Verification items for the finished model (mm, model axes). Face numbers are marked on the shaded views. A direction names the side the tool comes from. Coordinates: 2 decimals unless noted, no trailing zeros. Order: outer loops, then holes, each group sorted by start corner. A loop starts at its lowest first (then second) coordinate and runs counter-clockwise, first axis right, second up. Notation, with made-up numbers: M -2,-7.5 L 31,-7.5 A12 ccw 31,-1.5 Z; hole C 70,10.25 d8. An arc over 180 degrees is marked long. Write item = value, one per line.
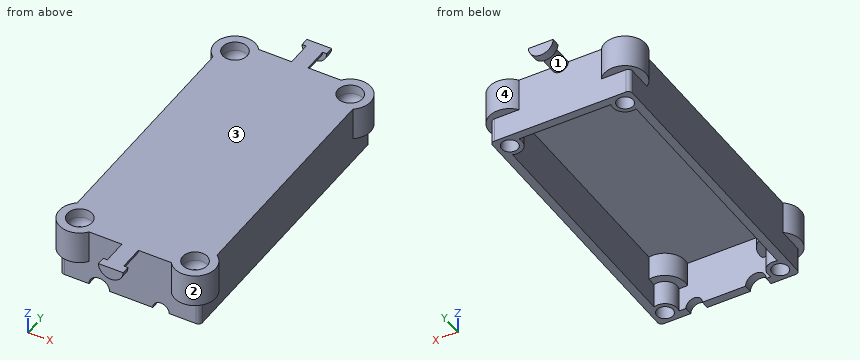
```python
from build123d import *

# Parameters (mm, degrees)
SKETCH1_W           = 34
SKETCH1_H           = 70
BOSS_EXTRUDE1_DEPTH = 14
SKETCH2_W           = 30
SKETCH2_H           = 66
CUT_EXTRUDE1_DEPTH  = 12
SKETCH3_R           = 3
BOSS_EXTRUDE2_DEPTH = 12
SKETCH4_R           = 2
CUT_EXTRUDE2_DEPTH  = 80.069589603
CUT_EXTRUDE4_REACH  = 81.07
SKETCH6_R           = 2.5
SKETCH6_R_2         = 2
FILLET1_R           = 1
BOSS_EXTRUDE3_START = -8
SKETCH7_R           = 5
SKETCH7_R_2         = 3
BOSS_EXTRUDE3_DEPTH = 8
CUT_EXTRUDE7_START  = -4
SKETCH8_R           = 3
CUT_EXTRUDE7_DEPTH  = 4
BOSS_EXTRUDE4_DEPTH = 8
CUT_EXTRUDE8_START  = -8
CUT_EXTRUDE8_DEPTH  = 6
BOSS_EXTRUDE5_START = 8
BOSS_EXTRUDE5_DEPTH = 8
CUT_EXTRUDE9_START  = -2
CUT_EXTRUDE9_DEPTH  = 6
FILLET3_R           = 2


with BuildPart() as part:
    # Sketch1 → Boss-Extrude1 (new body)
    with BuildSketch(Plane.XY):
        with Locations((17, 35)):
            Rectangle(SKETCH1_W, SKETCH1_H)
    extrude(amount=BOSS_EXTRUDE1_DEPTH)

    # Sketch2 → Cut-Extrude1 (cut)
    with BuildSketch(Plane(origin=(0, 0, 0), x_dir=(-1, 0, 0), z_dir=(0, 0, -1))):
        with Locations((-17, 35)):
            Rectangle(SKETCH2_W, SKETCH2_H)
    extrude(amount=-CUT_EXTRUDE1_DEPTH, mode=Mode.SUBTRACT)

    # Sketch3 → Boss-Extrude2 (add)
    with BuildSketch(Plane(origin=(0, 0, 0), x_dir=(-1, 0, 0), z_dir=(0, 0, -1))):
        with Locations((-31, 67)):
            Circle(SKETCH3_R)
        with Locations((-3, 67)):
            Circle(SKETCH3_R)
        with Locations((-3, 3)):
            Circle(SKETCH3_R)
        with Locations((-31, 3)):
            Circle(SKETCH3_R)
    extrude(amount=-BOSS_EXTRUDE2_DEPTH)

    # Sketch4 → Cut-Extrude2 (cut, through all)
    with BuildSketch(Plane(origin=(0, 0, 0), x_dir=(-1, 0, 0), z_dir=(0, 0, -1))):
        with Locations((-3, 67)):
            Circle(SKETCH4_R)
        with Locations((-31, 67)):
            Circle(SKETCH4_R)
        with Locations((-3, 3)):
            Circle(SKETCH4_R)
        with Locations((-31, 3)):
            Circle(SKETCH4_R)
    extrude(amount=-CUT_EXTRUDE2_DEPTH, mode=Mode.SUBTRACT)

    # Sketch6 → Cut-Extrude4 (cut, up to next)
    with BuildSketch(Plane.XZ, mode=Mode.PRIVATE) as cut_extrude4_sk1:
        with Locations((9.5, 0)):
            Circle(SKETCH6_R)
    cut_extrude4_tool1 = extrude(cut_extrude4_sk1.sketch, amount=-CUT_EXTRUDE4_REACH, mode=Mode.PRIVATE) & part.part
    # Sketch6 → Cut-Extrude4 (cut, up to next)
    with BuildSketch(Plane.XZ, mode=Mode.PRIVATE) as cut_extrude4_sk2:
        with Locations((24.5, 0)):
            Circle(SKETCH6_R_2)
    cut_extrude4_tool2 = extrude(cut_extrude4_sk2.sketch, amount=-CUT_EXTRUDE4_REACH, mode=Mode.PRIVATE) & part.part
    add(cut_extrude4_tool1.solids().sort_by_distance((9.5, 0, 0))[0], mode=Mode.SUBTRACT)
    add(cut_extrude4_tool2.solids().sort_by_distance((24.5, 0, 0))[0], mode=Mode.SUBTRACT)

    # Fillet1
    fillet1_edges = [part.edges().sort_by_distance(p)[0] for p in [
        (0, 70, 7),
        (34, 70, 7),
        (34, 0, 7),
        (0, 0, 7),
    ]]
    fillet(fillet1_edges, radius=FILLET1_R)

    # Sketch7 → Boss-Extrude3 (add)
    # profile 1 of 4: a face of its own
    with BuildSketch(Plane.XY.offset(14).offset(BOSS_EXTRUDE3_START)):
        with Locations((31, 67)):
            Circle(SKETCH7_R)
        with Locations((31, 67)):
            Circle(SKETCH7_R_2, mode=Mode.SUBTRACT)
    # profile 2 of 4: a face of its own
    with BuildSketch(Plane.XY.offset(14).offset(BOSS_EXTRUDE3_START)):
        with Locations((3, 67)):
            Circle(SKETCH7_R)
        with Locations((3, 67)):
            Circle(SKETCH7_R_2, mode=Mode.SUBTRACT)
    # profile 3 of 4: a face of its own
    with BuildSketch(Plane.XY.offset(14).offset(BOSS_EXTRUDE3_START)):
        with Locations((31, 3)):
            Circle(SKETCH7_R)
        with Locations((31, 3)):
            Circle(SKETCH7_R_2, mode=Mode.SUBTRACT)
    # profile 4 of 4: a face of its own
    with BuildSketch(Plane.XY.offset(14).offset(BOSS_EXTRUDE3_START)):
        with Locations((3, 3)):
            Circle(SKETCH7_R)
        with Locations((3, 3)):
            Circle(SKETCH7_R_2, mode=Mode.SUBTRACT)
    extrude(amount=BOSS_EXTRUDE3_DEPTH)

    # Sketch8 → Cut-Extrude7 (cut)
    with BuildSketch(Plane.XY.offset(14).offset(CUT_EXTRUDE7_START)):
        with Locations((3, 3)):
            Circle(SKETCH8_R)
        with Locations((31, 3)):
            Circle(SKETCH8_R)
        with Locations((31, 67)):
            Circle(SKETCH8_R)
        with Locations((3, 67)):
            Circle(SKETCH8_R)
    extrude(amount=CUT_EXTRUDE7_DEPTH, mode=Mode.SUBTRACT)

    # Sketch9 → Boss-Extrude4 (add)
    with BuildSketch(Plane(origin=(0, 70, 0), x_dir=(1, 0, 0), z_dir=(0, 1, 0))):
        with BuildLine():
            Line((20, -14), (14, -14))
            ThreePointArc((14, -14), (17, -11), (20, -14))
        make_face()
    extrude(amount=BOSS_EXTRUDE4_DEPTH)

    # Sketch10 → Cut-Extrude8 (cut)
    with BuildSketch(Plane(origin=(0, 78, 0), x_dir=(1, 0, 0), z_dir=(0, 1, 0)).offset(CUT_EXTRUDE8_START)):
        with BuildLine():
            Line((19, -14), (20, -14))
            ThreePointArc((20, -14), (17, -11), (14, -14))
            Line((14, -14), (15, -14))
            ThreePointArc((15, -14), (17, -12), (19, -14))
        make_face()
    extrude(amount=CUT_EXTRUDE8_DEPTH, mode=Mode.SUBTRACT)

    # Sketch11 → Boss-Extrude5 (add)
    with BuildSketch(Plane.XZ.offset(BOSS_EXTRUDE5_START)):
        with BuildLine():
            Line((20, 14), (14, 14))
            ThreePointArc((14, 14), (17, 11), (20, 14))
        make_face()
    extrude(amount=-BOSS_EXTRUDE5_DEPTH)

    # Sketch12 → Cut-Extrude9 (cut)
    with BuildSketch(Plane.XZ.offset(8).offset(CUT_EXTRUDE9_START)):
        with BuildLine():
            Line((14, 14), (15, 14))
            ThreePointArc((15, 14), (17, 12), (19, 14))
            Line((19, 14), (20, 14))
            ThreePointArc((20, 14), (17, 11), (14, 14))
        make_face()
    extrude(amount=-CUT_EXTRUDE9_DEPTH, mode=Mode.SUBTRACT)

    # Fillet3
    # the kernel refuses this fillet: 2 mm, written as the material it adds along each edge
    with BuildSketch(Plane(origin=(3, 67, 10), x_dir=(1, 0, 0), z_dir=(0, -1, 0))) as fillet3_piece_1_section:
        with BuildLine():
            CenterArc((1, 1.732050808), FILLET3_R, 300, 60)
            Line((2, 0), (2.02, -0.034641016))
            ThreePointArc((2.02, -0.034641016), (2.5, -0.04), (3, -0.04))
            Line((3, -0.04), (3.04, 0))
            Line((3.04, 0), (3.04, 1.732050808))
            Line((3.04, 1.732050808), (3, 1.732050808))
        make_face()
    fillet3_piece_1 = revolve(axis=Axis((3, 67, 10), (0, 0, 1)), mode=Mode.PRIVATE)
    fillet3_piece_1 = fillet3_piece_1 - Plane(origin=(3, 67, 10.721085361), x_dir=(-1, 0, 0), z_dir=(0, 0, -1)) * Cylinder(2, 13, mode=Mode.PRIVATE)
    add(fillet3_piece_1)
    with BuildSketch(Plane(origin=(31, 67, 10), x_dir=(1, 0, 0), z_dir=(0, -1, 0))) as fillet3_piece_2_section:
        with BuildLine():
            CenterArc((1, 1.732050808), FILLET3_R, 300, 60)
            Line((2, 0), (2.02, -0.034641016))
            ThreePointArc((2.02, -0.034641016), (2.5, -0.04), (3, -0.04))
            Line((3, -0.04), (3.04, 0))
            Line((3.04, 0), (3.04, 1.732050808))
            Line((3.04, 1.732050808), (3, 1.732050808))
        make_face()
    fillet3_piece_2 = revolve(axis=Axis((31, 67, 10), (0, 0, 1)), mode=Mode.PRIVATE)
    fillet3_piece_2 = fillet3_piece_2 - Plane(origin=(31, 67, 10.721085361), x_dir=(-1, 0, 0), z_dir=(0, 0, -1)) * Cylinder(2, 13, mode=Mode.PRIVATE)
    add(fillet3_piece_2)
    with BuildSketch(Plane(origin=(31, 3, 10), x_dir=(1, 0, 0), z_dir=(0, -1, 0))) as fillet3_piece_3_section:
        with BuildLine():
            CenterArc((1, 1.732050808), FILLET3_R, 300, 60)
            Line((2, 0), (2.02, -0.034641016))
            ThreePointArc((2.02, -0.034641016), (2.5, -0.04), (3, -0.04))
            Line((3, -0.04), (3.04, 0))
            Line((3.04, 0), (3.04, 1.732050808))
            Line((3.04, 1.732050808), (3, 1.732050808))
        make_face()
    fillet3_piece_3 = revolve(axis=Axis((31, 3, 10), (0, 0, 1)), mode=Mode.PRIVATE)
    fillet3_piece_3 = fillet3_piece_3 - Plane(origin=(31, 3, 10.721085361), x_dir=(-1, 0, 0), z_dir=(0, 0, -1)) * Cylinder(2, 13, mode=Mode.PRIVATE)
    add(fillet3_piece_3)
    with BuildSketch(Plane(origin=(3, 3, 10), x_dir=(1, 0, 0), z_dir=(0, -1, 0))) as fillet3_piece_4_section:
        with BuildLine():
            CenterArc((1, 1.732050808), FILLET3_R, 300, 60)
            Line((2, 0), (2.02, -0.034641016))
            ThreePointArc((2.02, -0.034641016), (2.5, -0.04), (3, -0.04))
            Line((3, -0.04), (3.04, 0))
            Line((3.04, 0), (3.04, 1.732050808))
            Line((3.04, 1.732050808), (3, 1.732050808))
        make_face()
    fillet3_piece_4 = revolve(axis=Axis((3, 3, 10), (0, 0, 1)), mode=Mode.PRIVATE)
    fillet3_piece_4 = fillet3_piece_4 - Plane(origin=(3, 3, 10.721085361), x_dir=(-1, 0, 0), z_dir=(0, 0, -1)) * Cylinder(2, 13, mode=Mode.PRIVATE)
    add(fillet3_piece_4)


solid = part.part
```
Item 1: Sectioned sample at D-D, the plane y = 52. Enter the section's corners in (x, z).
Report:
outline = M 0,0 L 2,0 L 2,12 L 32,12 L 32,0 L 34,0 L 34,14 L 0,14 Z
Item 2: Sectioned sample at A-A, the plane z = 4.5. Enter the section's corners in (x, y).
Report:
outline = M 0,1 A1 ccw 1,0 L 33,0 A1 ccw 34,1 L 34,69 A1 ccw 33,70 L 1,70 A1 ccw 0,69 Z; hole C 3,3 d4; hole C 3,67 d4; hole M 2,5.83 A3 cw 5.83,2 L 28.17,2 A3 cw 32,5.83 L 32,64.17 A3 cw 28.17,68 L 5.83,68 A3 cw 2,64.17 Z; hole C 31,3 d4; hole C 31,67 d4
Item 3: Tool access check on the marked faces 1 and 2. Record the directions out of +Z, -Z, +X, -X, +Y, -Y that give a thin tool (end or side, any length) a straight path to the whole face; none if there is none.
Report:
face_1 = -Z
face_2 = +Z, -Z
Item 4: Gauge pin test, flat ends, axial feed: pin 1 (3 mm diameter, centred on x = 6.5, y = 64, fed in from -Z); pin 2 (3 mm diameter, centred on y = 8.5, z = 2.5, fed in from -X); pin 3 (3.5 mm diameter, centred on x = 22, z = 4.5, fed in from -Y). Record the tip position at first contact, or that the pin passes through.
Report:
pin_1 = 6
pin_2 = 0
pin_3 = 0
Item 5: Release check for a two-part mould opening along Y. For the marked faces 3 and 4 record: pulls with the +Y half, pulls with the -Y half, needs draft (parallel to the pull), parting line crosses it, or undercut.
Report:
face_3 = needs draft
face_4 = undercut
Item 6: Scan lines: L1, parallel to X at y = 3, z = 5; L2, parallel to Y at x = 3, z = 6.5; L3, parallel to X at y = 3, z = 7.75. Record each from-to range of solid material in increasing order. Write a range as from..to.
Report:
L1 = 0..1, 5..6, 28..29, 33..34
L2 = -2..1, 5..8, 62..65, 69..72
L3 = -2..1, 5..8, 26..29, 33..36
Item 7: Sectioned sample at C-C, the plane x = 24.5. Enter the section's corners in (y, z), then the cut area to 3 significant figures.
Report:
outline = M 0,2 L 2,2 L 2,12 L 68,12 L 68,0 L 70,0 L 70,14 L 0,14 Z
area = 184 mm^2
Item 8: Sectioned sample at B-B, the plane z = 1. Enter the section's corners in (x, y), then the cut area to 3 significant figures.
Report:
outline = M 0,1 A1 ccw 1,0 L 7.21,0 L 7.21,2 L 5.83,2 A3 ccw 2,5.83 L 2,64.17 A3 ccw 5.83,68 L 28.17,68 A3 ccw 32,64.17 L 32,5.83 A3 ccw 28.17,2 L 26.23,2 L 26.23,0 L 33,0 A1 ccw 34,1 L 34,69 A1 ccw 33,70 L 1,70 A1 ccw 0,69 Z; M 11.79,0 L 22.77,0 L 22.77,2 L 11.79,2 Z; hole C 3,3 d4; hole C 3,67 d4; hole C 31,3 d4; hole C 31,67 d4
area = 389 mm^2
